```python
from build123d import *

# Parameters (mm, degrees)
SKETCH1_R           = 8.25
BOSS_EXTRUDE1_DEPTH = 3
SKETCH2_W           = 17.25
SKETCH2_H           = 3
BOSS_EXTRUDE2_DEPTH = 5
BOSS_EXTRUDE3_DEPTH = 3
SKETCH4_R           = 2.75
SKETCH4_R_2         = 0.6
CUT_EXTRUDE1_DEPTH  = 55.313902456


with BuildPart() as part:
    # Sketch1 → Boss-Extrude1 (new body)
    # profile 1 of 2: a face of its own
    with BuildSketch(Plane.XY):
        with BuildLine():
            Line((-3.25, 0), (0, 0))
            Line((0, 0), (0, 10))
            Line((0, 10), (-2.75, 10))
            ThreePointArc((-2.75, 10), (-4.517766953, 10.732233047), (-5.25, 12.5))
            Line((-5.25, 12.5), (-5.25, 15.5))
            Line((-5.25, 15.5), (-23, 15.5))
            Line((-23, 15.5), (-23, -20.5))
            Line((-23, -20.5), (-5.75, -20.5))
            Line((-5.75, -20.5), (-5.75, -2.5))
            ThreePointArc((-5.75, -2.5), (-5.017766953, -0.732233047), (-3.25, 0))
        make_face()
        with Locations((-13.08, 5)):
            Circle(SKETCH1_R, mode=Mode.SUBTRACT)
    # profile 2 of 2: a face of its own
    with BuildSketch(Plane.XY):
        with BuildLine():
            Line((0, 10), (0, 0))
            Line((0, 0), (3.25, 0))
            ThreePointArc((3.25, 0), (5.017766953, -0.732233047), (5.75, -2.5))
            Line((5.75, -2.5), (5.75, -20.5))
            Line((5.75, -20.5), (23, -20.5))
            Line((23, -20.5), (23, 15.5))
            Line((23, 15.5), (5.25, 15.5))
            Line((5.25, 15.5), (5.25, 12.5))
            ThreePointArc((5.25, 12.5), (4.517766953, 10.732233047), (2.75, 10))
            Line((2.75, 10), (0, 10))
        make_face()
        with Locations((13.08, 5)):
            Circle(SKETCH1_R, mode=Mode.SUBTRACT)
    extrude(amount=BOSS_EXTRUDE1_DEPTH)

    # Sketch2 → Boss-Extrude2 (add)
    # profile 1 of 2: a face of its own
    with BuildSketch(Plane.XZ.offset(20.5)):
        with BuildLine():
            Line((-23, 3), (-23, 0))
            Line((-23, 0), (-6, -24))
            ThreePointArc((-6, -24), (0, -30), (6, -24))
            Line((6, -24), (23, 0))
            Line((23, 0), (5.75, 0))
            Line((5.75, 0), (5.75, -5))
            Line((5.75, -5), (-5.75, -5))
            Line((-5.75, -5), (-5.75, 3))
            Line((-5.75, 3), (-23, 3))
        make_face()
        with BuildLine():
            Line((-3.449357744, -23.406762144), (-2.1, -7.6))
            ThreePointArc((-2.1, -7.6), (0, -5.5), (2.1, -7.6))
            Line((2.1, -7.6), (3.449357744, -23.406762144))
            ThreePointArc((3.449357744, -23.406762144), (3.487316454, -23.702302254), (3.5, -24))
            ThreePointArc((3.5, -24), (0, -27.5), (-3.5, -24))
            ThreePointArc((-3.5, -24), (-3.487316454, -23.702302254), (-3.449357744, -23.406762144))
        make_face(mode=Mode.SUBTRACT)
    # profile 2 of 2: a face of its own
    with BuildSketch(Plane.XZ.offset(20.5)):
        with Locations((14.375, 1.5)):
            Rectangle(SKETCH2_W, SKETCH2_H)
    extrude(amount=BOSS_EXTRUDE2_DEPTH)

    # Sketch3 → Boss-Extrude3 (add)
    with BuildSketch(Plane(origin=(0, -20.5, 0), x_dir=(1, 0, 0), z_dir=(0, 1, 0))):
        with BuildLine():
            Line((2.1, 7.6), (3.449357744, 23.406762144))
            ThreePointArc((3.449357744, 23.406762144), (0, 27.5), (-3.449357744, 23.406762144))
            Line((-3.449357744, 23.406762144), (-2.1, 7.6))
            ThreePointArc((-2.1, 7.6), (0, 5.5), (2.1, 7.6))
        make_face()
    extrude(amount=-BOSS_EXTRUDE3_DEPTH)

    # Sketch4 → Cut-Extrude1 (cut, through all)
    with BuildSketch(Plane.XZ.offset(23.5)):
        with Locations(Location((0, -24, 0), (0, 0, 270))):
            Circle(SKETCH4_R)
        with Locations(Location((0, -19.5, 0), (0, 0, 270))):
            Circle(SKETCH4_R_2)
        with Locations(Location((0, -16, 0), (0, 0, 270))):
            Circle(SKETCH4_R_2)
        with Locations(Location((0, -12.5, 0), (0, 0, 270))):
            Circle(SKETCH4_R_2)
        with Locations(Location((0, -9, 0), (0, 0, 270))):
            Circle(SKETCH4_R_2)
    extrude(amount=-CUT_EXTRUDE1_DEPTH, mode=Mode.SUBTRACT)


solid = part.part
```
Could you check a few things on this model? Use its own coordinates, in mm. A direction names the side the tool comes from. Round coordinates to 2 decimals unless told otherwise and drop trailing zeros. Loops run counter-clockwise (first coordinate to the right, second up) from the corner with the lowest first, then second, coordinate; pieces in that order, holes last. Notation, with made-up numbers: (44, 2) - (57, 2) arc R12 cw to (57, 24) - close; hole circle Ø4 at (32, 69). An arc over 180 degrees is marked (long way). Answer as CSV lines item,"result".
1. I want a section at D-D on z = -19.5. List the corners of the cut face in (x, y) for me, then the cut area to 3 significant figures.
Filled in:
outline,"(-9.19, -25.5) - (-3.12, -25.5) - (-3.12, -23.5) - (-0.6, -23.5) - (-0.6, -20.5) - (-9.19, -20.5) - close; (0.6, -23.5) - (3.12, -23.5) - (3.12, -25.5) - (9.19, -25.5) - (9.19, -20.5) - (0.6, -20.5) - close"
area,"75.8 mm^2"
2. On a 3-axis mill with a long thin cutter (end or side, diameter ignored), from which of +Z, -Z, +X, -X, +Y, -Y can I reach the whole of each face in a straight line? I mean faces 1 (the face through (0, -23.5, -17)), 2 (the face through (0, 2, 0)), 3 (the face through (4.998, -0.713, 1.479)). Say none if no direction works.
Filled in:
face 1,"-Y"
face 2,"-Z, +X, -X, +Y"
face 3,"+Z, -Z, -Y"
3. I want a section at A-A on y = 5. List the corners of the cut face in (x, z) for me.
Filled in:
outline,"(-23, 0) - (-21.33, 0) - (-21.33, 3) - (-23, 3) - close; (-4.83, 0) - (4.83, 0) - (4.83, 3) - (-4.83, 3) - close; (21.33, 0) - (23, 0) - (23, 3) - (21.33, 3) - close"
4. Please list where these lines run through material, in increasing order: line 1 along Y through (x, z) = (-13, 1); line 2 along X through (y, z) = (1, 0.5); line 3 along Y through (x, z) = (-16.5, -2). Write a range as [from, to].
Filled in:
line 1,"y = [-25.5, -3.25], [13.25, 15.5]"
line 2,"x = [-23, -20.3], [-5.86, 5.86], [20.3, 23]"
line 3,"y = [-25.5, -20.5]"
5. I want a section at C-C on x = -18. List the corners of the cut face in (y, z) for me, then the cut area to 3 significant figures.
Filled in:
outline,"(-25.5, -7.06) - (-20.5, -7.06) - (-20.5, 0) - (-1.62, 0) - (-1.62, 3) - (-25.5, 3) - close; (11.62, 0) - (15.5, 0) - (15.5, 3) - (11.62, 3) - close"
area,"119 mm^2"
6. We'd pull the mould along X, two halves only. Please class faces 4 (the face through (5.75, -16, 1)), 5 (the face through (-23, -5, 2)), 6 (the face through (14, 15.5, 1)): +X half, -X half, draft (parallel to the pull), parting line (faces both ways), or undercut.
Filled in:
face 4,"undercut"
face 5,"-X half"
face 6,"draft"
7. For pin 1 Ø2.5 at (y, z) = (-17.5, -1.5) entering from +X; pin 2 Ø15 at (x, z) = (-10, -12.5) entering from +Y; pin 3 Ø1.4 at (x, z) = (0, -19.5) entering from -Y; pin 4 Ø8 at (x, y) = (-8.5, -13.5) entering from -Z, each with a flat end and sliding along its axis, tell me the tip position at first contact or that it passes through.
Filled in:
pin 1,"passes through"
pin 2,"stops at y = -20.5"
pin 3,"stops at y = -23.5"
pin 4,"stops at z = 0"
8. I want a section at B-B on z = 1.5. List the corners of the cut face in (x, y) for me, then the cut area to 3 significant figures.
Filled in:
outline,"(-23, -25.5) - (-5.75, -25.5) - (-5.75, -2.5) arc R2.5 cw to (-3.25, 0) - (3.25, 0) arc R2.5 cw to (5.75, -2.5) - (5.75, -25.5) - (23, -25.5) - (23, 15.5) - (5.25, 15.5) - (5.25, 12.5) arc R2.5 cw to (2.75, 10) - (-2.75, 10) arc R2.5 cw to (-5.25, 12.5) - (-5.25, 15.5) - (-23, 15.5) - close; hole circle Ø16.5 at (-13.08, 5); hole circle Ø16.5 at (13.08, 5)"
area,"1,110 mm^2"
